from build123d import *

# Parameters (mm, degrees)
MODEL_R         = 4.5
MODEL_W         = 10
MODEL_H         = 2.2
EXTRUDE_1_DEPTH = 1


with BuildPart() as part:
    # Model → 凸台-拉伸1 (new body)
    with BuildSketch(Plane.XY):
        Polygon((4.28201841, 3.652217339), (4.28201841, 33.652217339), (6.28201841, 33.652217339), (6.28201841, 63.652217339), (4.28201841, 63.652217339), (4.28201841, 76.353862753), (53.28201841, 76.353862753), (53.28201841, 63.652217339), (51.28201841, 63.652217339), (51.28201841, 33.652217339), (53.28201841, 33.652217339), (53.28201841, 3.652217339), (34.53201841, 3.652217339), (34.53201841, 18.752217339), (28.78201841, 18.752217339), (23.03201841, 18.752217339), (23.03201841, 3.652217339), align=None)
        with Locations((28.78201841, 43.752217339)):
            Circle(MODEL_R, mode=Mode.SUBTRACT)
        with Locations((36.28201841, 28.925280735)):
            Rectangle(MODEL_W, MODEL_H, mode=Mode.SUBTRACT)
        with Locations((21.28201841, 28.925280735)):
            Rectangle(MODEL_W, MODEL_H, mode=Mode.SUBTRACT)
    extrude(amount=EXTRUDE_1_DEPTH)


solid = part.part
CAD build for the part. Positions are in the model's coordinates, mm. Give positions to 0.01 mm unless a question says otherwise; leave off trailing zeros. Loops run counter-clockwise (first coordinate to the right, second up) from the corner with the lowest first, then second, coordinate; pieces in that order, holes last. Notation, with made-up numbers: M -3,-29 L 26,-29 A32 cw 26,3 Z; hole C 43,-28 d10. An arc over 180 degrees is marked long. Write each question's results on one line, items separated by ' | '.
Q1. Flat gauge pin, fed straight in: P1, Ø10.5, axis at x = 28.78, y = 43.75, coming from the +Z side. Where does the tip first touch, or does it go through?
Geometry check:
P1: stops at z = 1
Q2. Probe probe 1 along Y at (x, z) = (39, 0.1); probe 2 along X at (y, z) = (17, 0.9); probe 3 along X at (y, z) = (53.5, 0.85). List the from-to ranges inside material, lowest first.
Geometry check:
probe 1: y = 3.65 to 27.83, 30.03 to 76.35 | probe 2: x = 4.28 to 23.03, 34.53 to 53.28 | probe 3: x = 6.28 to 51.28
Q3. Band-saw the part on A-A on x = 37.5. Write the cut outline in (y, z), and give its area (3 significant figures).
Geometry check:
outline: M 3.65,0 L 27.83,0 L 27.83,1 L 3.65,1 Z; M 30.03,0 L 76.35,0 L 76.35,1 L 30.03,1 Z | area: 70.5 mm²
Q4. Mould opens along Y. For faces 1 (the face through (28.196, 48.214, 0.493)), 2 (the face through (35, 41, 1)) say: pulls with the +Y half, pulls with the -Y half, needs draft (parallel to the pull), parting line crosses it, or undercut.
Geometry check:
face 1: undercut | face 2: needs draft
Q5. Band-saw the part on B-B on y = 11. Write the cut outline in (x, z).
Geometry check:
outline: M 4.28,0 L 23.03,0 L 23.03,1 L 4.28,1 Z; M 34.53,0 L 53.28,0 L 53.28,1 L 34.53,1 Z
Q6. Band-saw the part on D-D on y = 35.5. Write the cut outline in (x, z).
Geometry check:
outline: M 6.28,0 L 51.28,0 L 51.28,1 L 6.28,1 Z
Q7. Band-saw the part on C-C on z = 0.7. Write the cut outline in (x, y), and give its area (3 significant figures).
Geometry check:
outline: M 4.28,3.65 L 23.03,3.65 L 23.03,18.75 L 34.53,18.75 L 34.53,3.65 L 53.28,3.65 L 53.28,33.65 L 51.28,33.65 L 51.28,63.65 L 53.28,63.65 L 53.28,76.35 L 4.28,76.35 L 4.28,63.65 L 6.28,63.65 L 6.28,33.65 L 4.28,33.65 Z; hole M 16.28,27.83 L 26.28,27.83 L 26.28,30.03 L 16.28,30.03 Z; hole C 28.78,43.75 d9; hole M 31.28,27.83 L 41.28,27.83 L 41.28,30.03 L 31.28,30.03 Z | area: 3,160 mm²
